Part model, mm, in its own coordinate system. A direction names the side the tool comes from. Round coordinates to 2 decimals unless told otherwise and drop trailing zeros. Write each loop counter-clockwise with the first axis right and the second up, starting at its lowest first coordinate (ties: lowest second). Pieces come first, ordered by that corner, then holes. Notation, with made-up numbers: (-35, 31.5) -> (16, 31.5) arc R14 cw to (16, 38.5) -> close; hole circle Ø6 at (18.25, -7.75). An arc over 180 degrees is marked (long way). Return JSON: item names as keys, results as strings. Group by question number.
(1) Drop flat-ended pins along their axis: pin 1 Ø1 at (y, z) = (-0.5, -1) entering from +X; pin 2 Ø6 at (y, z) = (-4, 10.5) entering from -X; pin 3 Ø1 at (x, y) = (-11, 11) entering from +Z; pin 4 Ø1.5 at (x, y) = (-12, -3) entering from +Z. Give the stop position or say it passes through.
(2) Mould opens along Y. For faces 4 (the flat face through (-14, 0, -3)), 5 (the flat face through (6.488, -11.265, -1.479)), 6 (the flat face through (6.12, 12.6, -1.48)), 7 (the flat face through (7.85, -11.6, -1.48)) say: +Y half, -Y half, draft (parallel to the pull), parting line (faces both ways), or undercut.
(3) Tool access for faces 1 (the flat face through (-14, -1, -1)), 2 (the flat face through (7.865, 11.622, -1.479)), 3 (the flat face through (-14, 1, -1)): list every direction of +Z, -Z, +X, -X, +Y, -Y with a clear straight run to the whole face (end or side of a thin tool).
(4) Drill centre lines: L1, parallel to Z at x = -6.5, y = 9.5; L2, parallel to Z at x = 0, y = 7.75; L3, parallel to Y at x = 7.25, z = 6.5. Where is each one in solid material? Low to high. Write a range as from..to.
(5) Saw through at A-A (z = -0.75). List the corners of the cut face in (x, y), plus the area to 3 significant figures.
from build123d import *

# Parameters (mm, degrees)
F3_DEPTH = 3
F4_COUNT = 3


with BuildPart() as f1:
    # F0 (on Right) → F1 (revolve)
    with BuildSketch(Plane.YZ):
        with BuildLine():
            Line((-15, 0), (0, 0))
            Line((0, 0), (0, 25))
            ThreePointArc((0, 25), (-10.9011156317, 14.540669379), (-15, 0))
        make_face()
    revolve(axis=Axis((0, 0, 12.5), (0, 0, 1)))

    # F2 (on face) → F3 (join)
    with BuildSketch(Plane(origin=(0, 0, 0), x_dir=(1, 0, 0), z_dir=(0, 0, -1))):
        with BuildLine():
            Line((-13, 0), (-15, 0))
            ThreePointArc((-15, 0), (-14.9916550655, -0.5002783193), (-14.9666295471, -1))
            Line((-14.9666295471, -1), (-13, -1))
            Line((-13, -1), (-13, 0))
        make_face()
        with BuildLine():
            ThreePointArc((-14.9666295471, 1), (-14.9916550655, 0.5002783193), (-15, 0))
            Line((-15, 0), (-13, 0))
            Line((-13, 0), (-13, 1))
            Line((-13, 1), (-14.9666295471, 1))
        make_face()
    extrude(amount=F3_DEPTH)

    # F4: F1 ×3 about axis
    f4_axis = Axis((0, 0, 12.5), (0, 0, 1))


with BuildPart() as f1_1:
    add(f1.part)
    for i in range(1, F4_COUNT):
        add(f1.part.rotate(f4_axis, i * 360 / F4_COUNT))


solid = f1_1.part
Computed values:
{
 "1": {"pin 1": "x = -13", "pin 2": "x = -13.59", "pin 3": "through", "pin 4": "z = 13.27"},
 "2": {"face 4": "draft", "face 5": "undercut", "face 6": "+Y half", "face 7": "undercut"},
 "3": {"face 1": "-Z, +X, -X, -Y", "face 2": "-Z, +X", "face 3": "-Z, +X, -X, +Y"},
 "4": {"L1": "0..13.47", "L2": "0..18.83", "L3": "-12.2..12.2"},
 "5": {"outline": "(-14.97, -1) -> (-13, -1) -> (-13, 1) -> (-14.97, 1) arc R15 ccw to start; (5.63, -11.76) -> (6.62, -13.46) arc R15 ccw to (8.35, -12.46) -> (7.37, -10.76) -> close; (5.63, 11.76) -> (7.37, 10.76) -> (8.35, 12.46) arc R15 ccw to (6.62, 13.46) -> close", "area": "11.9 mm2"}
}
